Input: part model. Units: mm. Frame: model coordinates. Face numbers are marked on the shaded views. Round coordinates to 2 decimals unless told otherwise and drop trailing zeros. Order: outer loops, then holes, each group sorted by start corner. A loop starts at its lowest first (then second) coordinate and runs counter-clockwise, first axis right, second up. Notation, with made-up numbers: (66, 60.25) -> (76, 60.25) arc R9 cw to (76, 68.25) -> close; hole circle Ø3 at (67.25, 70). An arc over 180 degrees is marked (long way). Use a Markdown table: item, result.
from build123d import *

# Parameters (mm, degrees)
F0_R           = 16
F1_DEPTH       = 21
F3_D           = 6
F3_DEPTH       = 21
F3_CBORE_D     = 12
F3_CBORE_DEPTH = 12
F3_TIP         = 1.8025818571
F4_R           = 2


with BuildPart() as f1:
    # F0 (on Front) → F1 (new body)
    with BuildSketch(Plane.XZ):
        Circle(F0_R)
    extrude(amount=F1_DEPTH)

    # F3
    with Locations(Plane.XZ.offset(21)):
        with Locations((0, 0)):
            CounterBoreHole(F3_D / 2, F3_CBORE_D / 2, F3_CBORE_DEPTH, depth=F3_DEPTH)
            with Locations((0, 0, -(F3_DEPTH + F3_TIP / 2))):  # 118° drill point
                Cone(0, F3_D / 2, F3_TIP, mode=Mode.SUBTRACT)

    # F4
    f4_edges = [f1.edges().sort_by_distance(p)[0] for p in [
        (-16, -21, 0),
    ]]
    fillet(f4_edges, radius=F4_R)


solid = f1.part
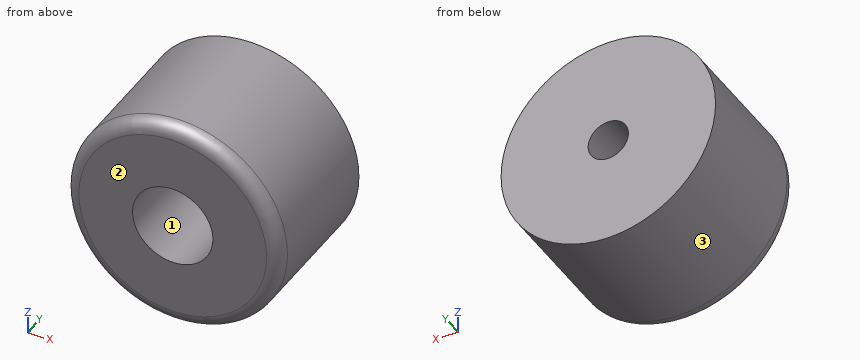
1) Cut plane C-C on y = -15. Return loops of the section in (x, z), and give its area (3 significant figures).
Results found:
| item | result |
|---|---|
| outline | circle Ø32 at (0, 0); hole circle Ø12 at (0, 0) |
| area | 691 mm² |
2) Line query: L1, parallel to Z at x = 0, y = -6.75; L2, parallel to Z at x = 0, y = -13.5; L3, parallel to X at y = -15, z = -3.5. Output: solid intervals per line, ascending. Write a range as [from, to].
Results found:
| item | result |
|---|---|
| L1 | z = [-16, -3], [3, 16] |
| L2 | z = [-16, -6], [6, 16] |
| L3 | x = [-15.61, -4.87], [4.87, 15.61] |
3) Pin query (flat end, axial travel): pin 1 Ø3.5 at (x, z) = (0.5, -2.5) entering from -Y; pin 2 Ø4 at (y, z) = (-9, 0.5) entering from +X; pin 3 Ø1 at (x, y) = (-3.5, -8.5) entering from +Z; pin 4 Ø2 at (y, z) = (-4, 3.5) entering from +X. Return the tip coordinate at first contact, or that it passes through.
Results found:
| item | result |
|---|---|
| pin 1 | stops at y = -9 |
| pin 2 | stops at x = 16 |
| pin 3 | stops at z = 15.72 |
| pin 4 | stops at x = 15.8 |
4) Cut plane A-A on z = 0. Return loops of the section in (x, y), and give its area (3 significant figures).
Results found:
| item | result |
|---|---|
| outline | (-16, -19) arc R2 ccw to (-14, -21) -> (-6, -21) -> (-6, -9) -> (-3, -9) -> (-3, 0) -> (-16, 0) -> close; (3, -9) -> (6, -9) -> (6, -21) -> (14, -21) arc R2 ccw to (16, -19) -> (16, 0) -> (3, 0) -> close |
| area | 472 mm² |
5) Pull-direction query (X, two-part tool) for the marked faces 1, 2 and 3; classes: +X half, -X half, draft (parallel to the pull), parting line (faces both ways), or undercut.
Results found:
| item | result |
|---|---|
| face 1 | undercut |
| face 2 | draft |
| face 3 | parting line |
6) Cut plane B-B on x = 0. Return loops of the section in (y, z), and give its area (3 significant figures).
Results found:
| item | result |
|---|---|
| outline | (-21, -14) arc R2 ccw to (-19, -16) -> (0, -16) -> (0, -3) -> (-9, -3) -> (-9, -6) -> (-21, -6) -> close; (-21, 6) -> (-9, 6) -> (-9, 3) -> (0, 3) -> (0, 16) -> (-19, 16) arc R2 ccw to (-21, 14) -> close |
| area | 472 mm² |
